Could you check a few things on this model? Use its own coordinates, in mm. A direction names the side the tool comes from. Round coordinates to 2 decimals unless told otherwise and drop trailing zeros. Write each loop counter-clockwise with the first axis right and the second up, starting at its lowest first coordinate (ties: lowest second). Pieces come first, ordered by that corner, then holes.
Autodesk Inventor part; units mm, degrees
ref_plane "Work Plane1" through (1.525, 0, 0) normal (0, 0, 1) x (1, 0, 0)
ref_plane "YZ Plane" through (0, 0, 0) normal (1, 0, 0) x (0, 1, 0)
ref_plane "XZ Plane" through (0, 0, 0) normal (0, 1, 0) x (-1, 0, 0)
sketch "Sketch1" plane through (0, 0, 0) normal (0, 0, 1) x (1, 0, 0)
  line L0 (0, 2.95) -> (0, 1.8106)
  line L1 (2.1, 2) -> (20, 2)
  line L2 (20, 2) -> (20, 0)
  line L3 (20, 0) -> (-0.4001, 0)
  line L4 (-4.4801, 0) -> (24.08, 0)
  line L5 (-0.4001, 0) -> (-0.4001, 2.95)
  line L6 (-0.4001, 2.95) -> (0, 2.95)
  line L7 (2.1, 2) -> (1.6705, 1.8106)
  line L8 (1.6705, 1.8106) -> (0, 1.8106)
  line L9 (0, -0.59) -> (0, 3.54)
  dimension "d0" = 20
  dimension "d1" = 17.9
  dimension "d2" = 4
  dimension "d9" = 0.4001
  dimension "d10" = 5.9
  dimension "d13" = 0.4295
  dimension "d14" = 3.6211
revolve "Body" add sketch "Sketch1" angle 360 about axis through (20, 0, 0) along (-1, 0, 0)
sketch "Sketch2" plane through (-0.4001, 0, 0) normal (-1, 0, 0) x (0, 0, 1)
  line L0 (0, 4.0415) -> (3.5, 2.0207)
  line L1 (3.5, 2.0207) -> (3.5, -2.0207)
  line L2 (3.5, -2.0207) -> (0, -4.0415)
  line L3 (0, -4.0415) -> (-3.5, -2.0207)
  line L4 (-3.5, -2.0207) -> (-3.5, 2.0207)
  line L5 (-3.5, 2.0207) -> (0, 4.0415)
  point P0 (0, 0)
  point P1 (0, 0)
  dimension "d11" = 7
extrude "Head" add sketch "Sketch2" along normal blind 2.4
sketch "Sketch4" plane through (0, 0, 0) normal (0, 0, 1) x (1, 0, 0)
  line L0 (-2.8001, 3.5) -> (-2.8001, 4.0415)
  line L1 (-2.8001, 4.0415) -> (-2.4875, 4.0415)
  line L2 (-2.4875, 4.0415) -> (-2.8001, 3.5)
  line L3 (-3.2801, 0) -> (0.0799, 0)
  line L4 (-0.4001, 4.0415) -> (-2.8001, 4.0415)
  line L5 (-2.8001, 2.0207) -> (-2.8001, 4.0415)
  dimension "d5" = 30
  dimension "d19" = 7
revolve "Chamfer1" cut sketch "Sketch4" angle 360 about axis through (-10, 0, 0) along (1, 0, 0)
thread "Thread"
chamfer "Chamfer2" distance 0.4294 distance2 0.4295 1 edges at (20, -2, 0) measured on face at (20, -0.5903, 0.3098)
ref_plane "Work Plane1" through (1.525, 0, 0) normal (0, 0, 1) x (1, 0, 0)
equation "\"d0\" = NLG"
equation "\"d1\" = GEL"
equation "\"d2\" = GD"
equation "\"d10\" = SD2"
equation "\"d14\" = BDM"
equation "\"d11\" = SW"
equation "\"d3\" = KOH - SD"
equation "\"d5\" = ANG1"
equation "\"d19\" = SW0"
equation "\"d15\" = GEL"
equation "\"d6\" = -0.5 * SPD + 0.5 * GD"
equation "\"NLG\" = 20"
equation "\"GD\" = NND"
equation "\"BDM\" = 3.62111"
equation "\"KOH\" = 2.8"
equation "\"GEL\" = 17.9"
equation "\"SW\" = 7"
equation "\"SW0\" = 7"
equation "\"SPD\" = NND - 1.2269 * PTC"
equation "\"SD2\" = 5.9"
equation "\"SD\" = 0.4"
equation "\"ANG1\" = 30deg"
equation "\"GAL\" = 0.61345 * PTC"
equation "\"GUL\" = 0.61345 * PTC"
equation "\"RR\" = 0.2"
equation "\"GD1\" = THREADDIA - 1.2269 * PTC"
equation "\"THREADDIA\" = 4"
equation "\"TOA\" = 30deg"
equation "\"PTC\" = 0.7"
equation "\"NND\" = 4"
equation "\"E0\" = 1.155 * SW"
properties part number "DIN 933 - M4  x 20" material "Steel, Mild"
Q1. Imagine slicing it at B-B, the plane x = 1. Write out the boundary of the cut face in (y, z), then the cut area to 3 significant figures.
Q2. On a 3-axis mill with a long thin cutter (end or side, diameter ignored), from which of +Z, -Z, +X, -X, +Y, -Y can I reach the whole of each face in a straight line? I mean faces 1 (the cylindrical face through (11, 0, -2)), 2 (the conical face through (-2.724, -3.632, 0.009)). Say none if no direction works.
Q3. Imagine slicing it at A-A, the plane x = 10. Write out the boundary of the cut face in (y, z).
Q4. I'm going to push flat-ended pins straight in: pin 1 Ø2 at (x, y) = (13.5, 2.5) entering from +Z; pin 2 Ø3 at (x, z) = (15.5, 2.5) entering from -Y; pin 3 Ø4 at (x, z) = (4, -1) entering from +Y. Where does each tip first touch, or does it pass through?
Q5. If I drill on L1, parallel to X at y = 2, z = 2.75; L2, parallel to X at y = -2.5, z = 1.5; L3, parallel to Z at x = 4.75, y = 1.25, over which ranges is the centre line in solid material (lowest first)?
Results found:
1. outline: circle Ø3.62 at (0, 0)
1. area: 10.3 mm2
2. face 1: +X
2. face 2: -X, -Y
3. outline: circle Ø4 at (0, 0)
4. pin 1: stops at z = 1.32
4. pin 2: stops at y = -1.73
4. pin 3: stops at y = 2
5. L1: x = -2.8 to -0.4
5. L2: x = -2.8 to 0
5. L3: z = -1.56 to 1.56
